Source: CAD feature listing. Evaluate the final solid. Frame: model axes, mm. Face numbers are marked on the shaded views. A direction names the side the tool comes from. Give positions to 0.01 mm unless a question says otherwise; leave off trailing zeros. Write each loop counter-clockwise with the first axis right and the second up, starting at its lowest first coordinate (ties: lowest second). Pieces come first, ordered by that corner, then holes. Notation, with made-up numbers: (32, -10.75) -> (67, -10.75) arc R6 ccw to (67, -6.75) -> close; hole circle Ø8 at (7.5, 34). An arc over 180 degrees is marked (long way). Answer as a JSON object with one key per item and string values. Group by question number.
Item 1: Section query B-B on z = 0. Give the number of separate pieces and of enclosed holes in the cut face, plus the area to 3 significant figures.
Item 2: Section query A-A on y = 2.25. Return the cut outline in (x, z) (1 decimal), plus the area to 3 significant figures.
Item 3: Access query for the marked faces 5, 6, 7, 8 and 9. Directions: +Z, -Z, +X, -X, +Y, -Y. A direction counts if a zero-diameter tool reaches every point of the face in a straight line with its end or side. Return the directions, or none.
Item 4: Section query C-C on x = 0. Return the cut outline in (y, z) (1 decimal).
Item 5: Ray query, probe 1 along X at (y, z) = (7.5, 0); probe 2 along Z at (x, y) = (0, 15.2) (3 decimals); probe 3 along X at (y, z) = (1.25, -0.5). Return the intervals inside material, ascending. Write a range as from..to.
Item 6: First-contact query: pin 1 Ø0.7 at (y, z) = (18, -0.5) entering from +X; pin 2 Ø1.6 at (x, z) = (0, 0) entering from +Y; pin 3 Ø3 at (y, z) = (4, -1) entering from -X. Flat tips, straight axial feed; report the tip coordinate or a pass-through.
Item 7: Pull-direction query (X, two-part tool) for the marked faces 1, 2, 3 and 4; classes: pulls with the +X half, pulls with the -X half, needs draft (parallel to the pull), parting line crosses it, or undercut.
Item 8: Section query D-D on y = 15.25. Return the cut outline in (x, z) (3 decimals), plus the area to 3 significant figures.
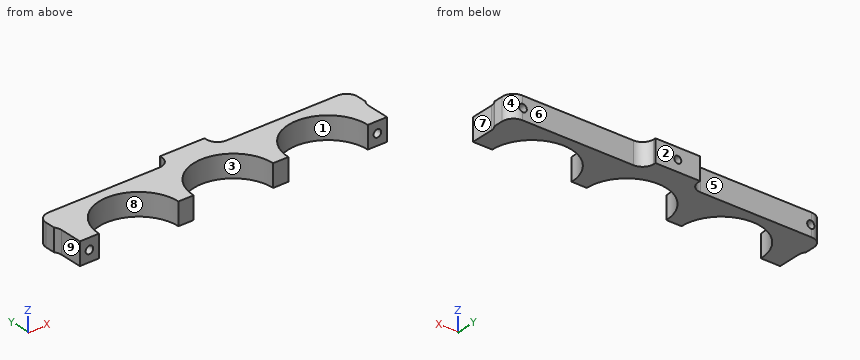
Autodesk Inventor part; units mm, degrees
ref_plane "YZ Plane" through (0, 0, 0) normal (1, 0, 0) x (0, 1, 0)
ref_plane "XZ Plane" through (0, 0, 0) normal (0, 1, 0) x (-1, 0, 0)
ref_plane "XY Plane" through (0, 0, 0) normal (0, 0, 1) x (1, 0, 0)
sketch "Sketch1" plane through (0, 0, 0) normal (0, 0, 1) x (1, 0, 0)
  line L0 (-44.323, 14.2875) -> (44.323, 14.2875)
  line L1 (44.323, 14.2875) -> (44.323, -14.2875)
  line L2 (44.323, -14.2875) -> (-44.323, -14.2875)
  line L3 (-44.323, -14.2875) -> (-44.323, 14.2875)
  point P0 (0, 0)
  dimension "d0" = 88.646
  dimension "d1" = 44.323
  dimension "d2" = 14.2875
  dimension "d3" = 28.575
extrude "Extrusion1" add sketch "Sketch1" along normal mid plane 6.35
sketch "Sketch2" plane through (0, 0, 3.175) normal (0, 0, 1) x (1, 0, 0)
  circle A0 centre (-26.924, 0) radius 11.303
  circle A1 centre (0, 0) radius 11.303
  line L0 (44.323, -14.2875) -> (44.323, 14.2875)
  circle A2 centre (26.924, 0) radius 11.303
  line L1 (-44.323, 14.2875) -> (-44.323, -14.2875)
  line L2 (-44.323, 0) -> (44.323, 0) construction
  line L3 (44.323, 14.2875) -> (-44.323, 14.2875)
  point P0 (0, 0)
  dimension "d6" = 22.606
  dimension "d9" = 22.606
  dimension "d11" = 22.606
  dimension "d14" = 26.924
  dimension "d21" = 88.646
  dimension "d22" = 26.924
  dimension "d45" = 0
sketch "Sketch4" plane through (-44.323, -14.2875, -3.175) normal (-1, 0, 0) x (0, 0, 1)
  line L0 (0, 0) -> (0, 28.575)
  line L1 (6.35, 28.575) -> (6.35, 0)
  line L2 (0, 22.6695) -> (6.35, 22.6695)
  line L3 (6.35, 22.6695) -> (6.35, 5.9055)
  line L4 (6.35, 5.9055) -> (0, 5.9055)
  line L5 (0, 5.9055) -> (0, 22.6695)
  point P0 (3.175, 14.2875)
  dimension "d30" = 8.382
  dimension "d31" = 16.764
extrude "Extrusion3" cut sketch "Sketch4" against normal blind 0.635
mirror "Mirror1" about plane through (0, 0, 0) normal (1, 0, 0) of "Extrusion3"
sketch "Sketch7" plane through (-44.323, -14.2875, 3.175) normal (0, -1, 0) x (1, 0, 0)
  line L0 (30.353, -14.605) -> (58.293, -14.605)
  line L1 (58.293, -14.605) -> (58.293, 8.255)
  line L2 (58.293, 8.255) -> (30.353, 8.255)
  line L3 (30.353, 8.255) -> (30.353, -14.605)
  point P0 (44.323, -3.175)
  dimension "d39" = 27.94
  dimension "d40" = 22.86
  dimension "d41" = 11.43
  dimension "d42" = 13.97
extrude "Extrusion5" [suppressed]
extrude "Extrusion6" cut sketch "Sketch2" against normal blind 25.4
sketch "Sketch8" plane through (0, 0, -3.175) normal (0, 0, -1) x (-1, 0, 0)
  line L0 (43.688, 8.382) -> (43.688, -8.382) construction
  line L1 (43.688, 0) -> (-43.688, 0)
  line L2 (-43.688, 8.382) -> (-43.688, -8.382) construction
  line L3 (44.323, 14.2875) -> (-44.323, 14.2875)
  line L4 (44.323, 8.382) -> (44.323, 14.2875)
  line L5 (-44.323, 14.2875) -> (-44.323, 8.382)
  line L6 (-43.688, 8.382) -> (-43.688, 0)
  line L7 (-44.323, 8.382) -> (-43.688, 8.382)
  line L8 (43.688, 8.382) -> (43.688, 0)
  line L9 (43.688, 8.382) -> (44.323, 8.382)
  point P0 (0, 0)
extrude "Extrusion7" [suppressed]
sketch "Sketch9" plane through (0, 0, -3.175) normal (0, 0, -1) x (-1, 0, 0)
  line L0 (-44.323, -14.2875) -> (44.323, -14.2875)
  line L1 (44.323, -14.2875) -> (44.323, -8.382)
  line L2 (44.323, -8.382) -> (43.688, -8.382)
  line L3 (-43.688, -8.382) -> (-44.323, -8.382)
  line L4 (-44.323, -8.382) -> (-44.323, -14.2875)
  line L5 (-43.688, 8.382) -> (-43.688, -8.382)
  line L6 (-43.688, 0) -> (-43.688, -8.382)
  line L7 (-43.688, 0) -> (43.688, 0)
  line L8 (43.688, -8.382) -> (43.688, 8.382)
  line L9 (43.688, -8.382) -> (43.688, 0)
  point P0 (0, 0)
extrude "Extrusion8" cut sketch "Sketch9" against normal through all
fillet "Fillet1" radius 3.175 2 edges at (-44.323, 14.2875, 0) (44.323, 14.2875, 0)
sketch "Sketch12" plane through (-41.148, 14.2875, -3.175) normal (0, 1, 0) x (1, 0, 0)
  line L0 (82.296, -6.35) -> (0, -6.35)
  line L1 (34.798, 0) -> (47.498, 0)
  line L2 (47.498, 0) -> (47.498, -6.35)
  line L3 (47.498, -6.35) -> (34.798, -6.35)
  line L4 (34.798, -6.35) -> (34.798, 0)
  circle A0 centre (41.148, -3.175) radius 1
  line L5 (29.845, 0) -> (52.451, 0)
  dimension "d81" = 6.35
  dimension "d82" = 12.7
  dimension "d83" = 2
  dimension "d87" = 0
extrude "Extrusion11" add sketch "Sketch12" along normal blind 3.8
fillet "Fillet3" radius 3.175 2 edges at (6.35, 14.2875, 0) (-6.35, 14.2875, 0)
thread "Thread3"
fillet "Fillet4" radius 3.175 2 edges at (43.688, 8.382, 0) (-43.688, 8.382, 0)
sketch "Sketch10" plane through (-43.688, 0, -3.175) normal (0, -1, 0) x (1, 0, 0)
  line L0 (5.461, 6.35) -> (5.461, 0)
  line L1 (0, 0) -> (0, 6.35)
  line L2 (-0.635, 0) -> (-0.635, 6.35)
  line L3 (5.461, 6.35) -> (5.461, 0)
  line L4 (0, 6.35) -> (5.461, 6.35)
  line L5 (0, 0) -> (0, 6.35)
  line L6 (5.461, 0) -> (0, 0)
  circle A0 centre (2.7305, 3.175) radius 1.5494
  line L7 (86.614, 1.27) -> (80.264, 1.27)
  line L8 (86.614, 0) -> (80.264, 0)
  point P0 (43.688, 3.175)
  point P1 (84.328, 1.27)
  point P2 (77.978, 1.27)
  point P3 (84.328, 0)
  point P4 (77.978, 0)
  dimension "d58" = 3.0988
  dimension "d61" = 5.461
  dimension "d62" = 2.7305
  dimension "d78" = 3.175
  dimension "d90" = 6.35
hole "Hole1" at (-40.9575, 0, 0) direction (0, 1, 0) diameter 2.159 end through all
mirror "Mirror3" about plane through (0, 0, 0) normal (1, 0, 0) of "Hole1"
equation "\"d9\" = d7"
equation "\"d11\" = d9"
equation "\"d22\" = d14"
equation "\"d62\" = 0.5 * d61"
equation "\"d78\" = 0.5 * d90"
equation "\"d7\" = d6"
properties part number "Tube Holder Halve 2" material "Aluminum 6061-AHC"
Worked answers:
{
 "1": {"separate pieces": "3", "enclosed holes": "0", "area": "634 mm^2"},
 "2": {"outline": "(-43.7, -3.2) -> (-38, -3.2) -> (-38, 3.2) -> (-43.7, 3.2) -> close; (-15.8, -3.2) -> (-11.1, -3.2) -> (-11.1, 3.2) -> (-15.8, 3.2) -> close; (11.1, -3.2) -> (15.8, -3.2) -> (15.8, 3.2) -> (11.1, 3.2) -> close; (38, -3.2) -> (43.7, -3.2) -> (43.7, 3.2) -> (38, 3.2) -> close; hole circle Ø2.2 at (-41, 0); hole circle Ø2.2 at (41, 0)", "area": "125 mm^2"},
 "3": {"face 5": "+Z, -Z, -X, +Y", "face 6": "+Z, -Z, +X, +Y", "face 7": "+Z, -Z, +X, -Y", "face 8": "+Z, -Z, -Y", "face 9": "+Z, -Z, -X, -Y"},
 "4": {"outline": "(11.3, -3.2) -> (18.1, -3.2) -> (18.1, -1) -> (14.3, -1) -> (14.3, 1) -> (18.1, 1) -> (18.1, 3.2) -> (11.3, 3.2) -> close"},
 "5": {"probe 1": "-43.86..-42.04, -39.88..-35.38, -18.47..-8.46, 8.46..18.47, 35.38..39.88, 42.04..43.86", "probe 2": "-3.175..-1, 1..3.175", "probe 3": "-43.69..-41.91, -40..-38.16, -15.69..-11.23, 11.23..15.69, 38.16..40, 41.91..43.69"},
 "6": {"pin 1": "x = 6.35", "pin 2": "y = 14.29", "pin 3": "x = -43.69"},
 "7": {"face 1": "undercut", "face 2": "needs draft", "face 3": "undercut", "face 4": "pulls with the +X half"},
 "8": {"outline": "(-7.248, -3.175) -> (7.248, -3.175) -> (7.248, 3.175) -> (-7.248, 3.175) -> close; hole circle Ø2 at (0, 0)", "area": "88.9 mm^2"}
}
